Autodesk Inventor part; units mm, degrees
ref_plane "Work Plane1" through (0, 0, 6) normal (0, 0, 1) x (1, 0, 0)
ref_plane "YZ Plane" through (0, 0, 0) normal (1, 0, 0) x (0, 1, 0)
ref_plane "XZ Plane" through (0, 0, 0) normal (0, 1, 0) x (-1, 0, 0)
sketch "Sketch1" plane through (0, 0, 0) normal (0, 1, 0) x (-1, 0, 0)
  circle A0 centre (0, 0) radius 6
  dimension "d0" = 12
extrude "Extrusion1" add sketch "Sketch1" against normal blind 8
chamfer "Chamfer1" distance 0.2 angle 45 2 edges at (6, -8, 0) (6, 0, 0)
sketch "Sketch2" plane through (0, -8, 0) normal (0, -1, 0) x (1, 0, 0)
  point P0 (0, 0)
hole "Hole1" at (0, -8, 0) direction (0, 1, 0) diameter 4 end through all
chamfer "Chamfer2" distance 0.2 angle 45 2 edges at (0, -8, 2) (0, 0, 2)
ref_plane "Work Plane1" through (0, 0, 6) normal (0, 0, 1) x (1, 0, 0)
sketch "Sketch3" plane through (0, 0, 6) normal (0, 0, 1) x (1, 0, 0)
  line L0 (-6, -0.2) -> (-6, -7.8)
  line L1 (-5.8, 0) -> (5.8, 0)
  point P0 (0, 0)
  point P1 (0, -4)
  point P2 (-6, -4)
hole "Hole2" at (0, -4, 6) direction (0, 0, -1) diameter 3.688 end up to surface
chamfer "Chamfer3" distance 0.2 angle 45 2 edges at (1.8366, -3.8348, 5.712) (-1.844, -4.0029, 5.7096)
properties part number "08-0003" material "Aluminum 6061"
Here's how the part is built. I have some questions about the finished solid (model axes, mm). Give positions to 0.01 mm unless a question says otherwise; leave off trailing zeros. Write each loop counter-clockwise with the first axis right and the second up, starting at its lowest first coordinate (ties: lowest second). Pieces come first, ordered by that corner, then holes. Notation, with made-up numbers: M -22,61 L 32,61 A14 cw 32,74 Z; hole C -16,0 d11. An arc over 180 degrees is marked long. Put each result on its own line as item: value. Start each with the question number.
Item 1: Will these pins go through, and if not, where does the flat tip stop? pin 1 (3 mm diameter, centred on y = -6, z = -2.5, fed in from +X); pin 2 (3 mm diameter, centred on y = -2.5, z = -4.5, fed in from -X); pin 3 (2 mm diameter, centred on y = -6.5, z = 3.5, fed in from -X).
Item 2: I need wall thicknesses on L1, parallel to Y at x = 0, z = 4.6; L2, parallel to Z at x = 0, y = -0.5; L3, parallel to Z at x = 0.75, y = -2.25. Which ranges of each line are inside material? Lowest first, please. Write a range as from..to.
Item 3: If we section it at A-A, the plane z = 0: Write out the boundary of the cut face in (x, y), then the cut area to 3 significant figures.
Item 4: Thinking about a two-plate mould opening in Z: for faces 1 (the cylindrical face through (1.301, -3.947, -5.857)), 2 (the cylindrical face through (0.766, -3.947, -1.847)), 3 (the cylindrical face through (-1.2, -2.6, 3.8)), which applies, +Z half, -Z half, draft (parallel to the pull), parting line (faces both ways), or undercut?
Item 5: If we section it at B-B, the plane x = 0: Count the separate pieces of the cut face and the enclosed holes in it, then the cut area to 3 significant figures.
Values:
1. pin 1: x = 5.92
1. pin 2: x = -5.2
1. pin 3: x = -5.45
2. L1: -8..-5.84, -2.16..0
2. L2: -6..-2, 2..6
2. L3: -5.95..-1.85, 1.85..5.81
3. outline: M -6,-7.8 L -5.8,-8 L -2.2,-8 L -2,-7.8 L -2,-0.2 L -2.2,0 L -5.8,0 L -6,-0.2 Z; M 2,-7.8 L 2.2,-8 L 5.8,-8 L 6,-7.8 L 6,-0.2 L 5.8,0 L 2.2,0 L 2,-0.2 Z
3. area: 63.8 mm²
4. face 1: parting line
4. face 2: undercut
4. face 3: draft
5. separate pieces: 3
5. enclosed holes: 0
5. area: 49.0 mm²
